Design review of the part built by this model. Coordinates are the model's own, in mm. Face numbers are marked on the shaded views. A direction names the side the tool comes from. Give positions to 0.01 mm unless a question says otherwise; leave off trailing zeros. Write each loop counter-clockwise with the first axis right and the second up, starting at its lowest first coordinate (ties: lowest second). Pieces come first, ordered by that corner, then holes. Notation, with made-up numbers: M 49,50.5 L 75,50.5 A34 ccw 75,80.5 Z; hole C 84,-10 d11. An arc over 180 degrees is marked long. Answer in a Markdown table with one row per item.
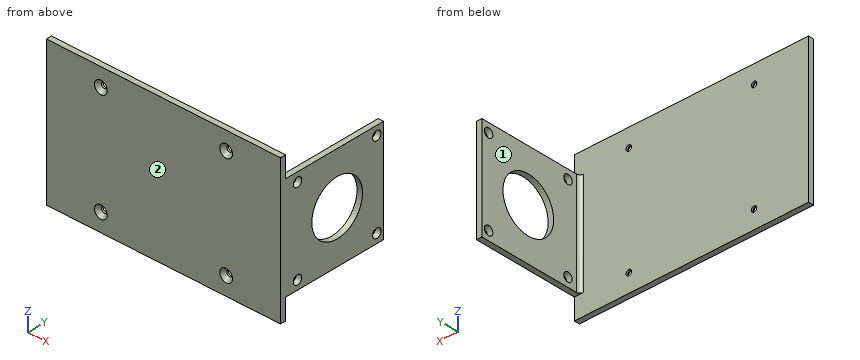
```python
from build123d import *

# Parameters (mm, degrees)
SKETCH1_W           = 129
SKETCH1_H           = 80
SKETCH1_R           = 1.5
BOSS_EXTRUDE1_DEPTH = 3
SKETCH2_W           = 3
SKETCH2_H           = 57
BOSS_EXTRUDE2_DEPTH = 58
FILLET1_R           = 2
SKETCH3_R           = 2.5
SKETCH3_R_2         = 15
CUT_EXTRUDE1_DEPTH  = 164.590953295
CHAMFER3_SIZE       = 2


with BuildPart() as part:
    # Sketch1 → Boss-Extrude1 (new body)
    with BuildSketch(Plane(origin=(0, 0, 0), x_dir=(1, 0, 0), z_dir=(0, 1, 0))):
        with Locations((64.5, 40)):
            Rectangle(SKETCH1_W, SKETCH1_H)
        with Locations(Location((99, 70, 0), (0, 0, 270))):
            Circle(SKETCH1_R, mode=Mode.SUBTRACT)
        with Locations(Location((30, 70, 0), (0, 0, 270))):
            Circle(SKETCH1_R, mode=Mode.SUBTRACT)
        with Locations(Location((99, 10, 0), (0, 0, 90))):
            Circle(SKETCH1_R, mode=Mode.SUBTRACT)
        with Locations(Location((30, 10, 0), (0, 0, 90))):
            Circle(SKETCH1_R, mode=Mode.SUBTRACT)
    extrude(amount=BOSS_EXTRUDE1_DEPTH)

    # Sketch2 → Boss-Extrude2 (add)
    with BuildSketch(Plane(origin=(0, 3, 0), x_dir=(1, 0, 0), z_dir=(0, 1, 0))):
        with Locations((127.5, 40)):
            Rectangle(SKETCH2_W, SKETCH2_H)
    extrude(amount=BOSS_EXTRUDE2_DEPTH)

    # Fillet1
    fillet1_edges = [part.edges().sort_by_distance(p)[0] for p in [
        (126, 3, -40),
    ]]
    fillet(fillet1_edges, radius=FILLET1_R)

    # Sketch3 → Cut-Extrude1 (cut, through all)
    with BuildSketch(Plane(origin=(129, 0, 0), x_dir=(0, 0, -1), z_dir=(1, 0, 0))):
        with Locations((16.5, 57)):
            Circle(SKETCH3_R)
        with Locations((40, 33.5)):
            Circle(SKETCH3_R_2)
        with Locations((63.5, 57)):
            Circle(SKETCH3_R)
        with Locations((16.5, 10)):
            Circle(SKETCH3_R)
        with Locations((63.5, 10)):
            Circle(SKETCH3_R)
    extrude(amount=-CUT_EXTRUDE1_DEPTH, mode=Mode.SUBTRACT)

    # Chamfer3
    chamfer3_edges = [part.edges().sort_by_distance(p)[0] for p in [
        (99, 0, -71.5),
        (30, 0, -71.5),
        (99, 0, -8.5),
        (30, 0, -8.5),
    ]]
    chamfer(chamfer3_edges, length=CHAMFER3_SIZE)


solid = part.part
```
1) Add section C-C (x = 30). Write out the cut boundary in (y, z), and give its area (3 significant figures).
Geometry says:
| item | result |
|---|---|
| outline | M 0,-80 L 3,-80 L 3,-71.5 L 2,-71.5 L 0,-73.5 Z; M 0,-66.5 L 2,-68.5 L 3,-68.5 L 3,-11.5 L 2,-11.5 L 0,-13.5 Z; M 0,-6.5 L 2,-8.5 L 3,-8.5 L 3,0 L 0,0 Z |
| area | 214 mm^2 |
2) For the marked faces 1 and 2, list the 3-axis set-ups (+Z, -Z, +X, -X, +Y, -Y) from which the entire face can be reached by the end or side of a thin tool; tool diameter is ignored.
Geometry says:
| item | result |
|---|---|
| face 1 | +Z, -Z, -X, +Y |
| face 2 | +Z, -Z, +X, -X, -Y |
3) Add section B-B (z = -16.5). Write out the cut boundary in (x, y).
Geometry says:
| item | result |
|---|---|
| outline | M 0,0 L 129,0 L 129,7.5 L 126,7.5 L 126,5 A2 cw 124,3 L 0,3 Z; M 126,12.5 L 129,12.5 L 129,54.5 L 126,54.5 Z; M 126,59.5 L 129,59.5 L 129,61 L 126,61 Z |
4) Insertion check: P1, Ø12, axis at x = 92, z = -66, coming from the +Y side; P2, Ø5, axis at x = 99, z = -10, coming from the -Y side; P3, Ø12, axis at y = 21, z = -40.5, coming from the -X side. Each pin has a flat end and moves straight along its axis. Give the tip position at first contact, or say it passes through.
Geometry says:
| item | result |
|---|---|
| P1 | y = 3 |
| P2 | y = 1 |
| P3 | x = 126 |
5) Add section A-A (y = 57). Write out the cut boundary in (x, z).
Geometry says:
| item | result |
|---|---|
| outline | M 126,-68.5 L 129,-68.5 L 129,-66 L 126,-66 Z; M 126,-61 L 129,-61 L 129,-19 L 126,-19 Z; M 126,-14 L 129,-14 L 129,-11.5 L 126,-11.5 Z |
6) To check wall thickness, follow probe 1 along Y at (x, z) = (128.1, -16.5); probe 2 along X at (y, z) = (2.35, -70); probe 3 along Y at (x, z) = (127, -16). State the ranges of each line that lie inside material, in increasing order. Write a range as [from, to].
Geometry says:
| item | result |
|---|---|
| probe 1 | [0, 7.5], [12.5, 54.5], [59.5, 61] |
| probe 2 | [0, 28.5], [31.5, 97.5], [100.5, 129] |
| probe 3 | [0, 7.55], [12.45, 54.55], [59.45, 61] |
7) Add section D-D (z = -40). Write out the cut boundary in (x, y).
Geometry says:
| item | result |
|---|---|
| outline | M 0,0 L 129,0 L 129,18.5 L 126,18.5 L 126,5 A2 cw 124,3 L 0,3 Z; M 126,48.5 L 129,48.5 L 129,61 L 126,61 Z |
